```python
from build123d import *

# Parameters (mm, degrees)
F0_R     = 12.5
F1_DEPTH = 5
F2_R     = 6.5
F3_DEPTH = 2.54
F4_DEPTH = 3
F5_R     = 6.5
F6_DEPTH = 3


with BuildPart() as f1:
    # F0 (on Top) → F1 (new body)
    with BuildSketch(Plane.XY):
        Circle(F0_R)
    extrude(amount=F1_DEPTH)

    # F2 (on Top) → F3 (join)
    with BuildSketch(Plane.XY):
        Circle(F2_R)
    extrude(amount=F3_DEPTH)

    # F2 (on Top) → F4 (join)
    with BuildSketch(Plane.XY):
        Circle(F2_R)
    extrude(amount=F4_DEPTH)

    # F5 (on Top) → F6 (cut)
    with BuildSketch(Plane.XY):
        Circle(F5_R)
    extrude(amount=F6_DEPTH, mode=Mode.SUBTRACT)


solid = f1.part
```
The model under review builds one solid part; all positions refer to its coordinate system, in mm. A direction names the side the tool comes from. Round coordinates to 2 decimals unless told otherwise and drop trailing zeros. Write each loop counter-clockwise with the first axis right and the second up, starting at its lowest first coordinate (ties: lowest second). Pieces come first, ordered by that corner, then holes.
(1) Machinability: for faces 4 (the flat face through (0, 0, 5)), 5 (the cylindrical face through (-5.158, -3.955, 1.479)), which of the approach directions +Z, -Z, +X, -X, +Y, -Y give a long, thin tool a straight path to every point of the face, cutting with its end or side? Answer none if there is none.
(2) We need section D-D on z = 3.35. Give the boundary of the cut face in (x, y), and give its area (3 significant figures).
(3) Wall thickness on L1, parallel to Y at x = 0, z = 1.3; L2, parallel to Z at x = 5.25, y = -2; L3, parallel to X at y = 5.75, z = 2.5: over which ranges is each line inside the solid? List them lowest first.
(4) Mouldability with a two-part tool opening along X and no side actions: class faces 1 (the cylindrical face through (11.923, 3.755, 2.465)), 2 (the flat face through (0, 0, 3)), 3 (the flat face through (5, -5, 0)) as +X half, -X half, draft (parallel to the pull), parting line (faces both ways), or undercut.
(5) We need section C-C on z = 0.4. Give the boundary of the cut face in (x, y).
(6) Insertion check: pin 1 (3 mm diameter, centred on y = -6.5, z = 3.5, fed in from -X); pin 2 (3 mm diameter, centred on y = -3.5, z = 2.5, fed in from +X); pin 3 (4 mm diameter, centred on x = 0, y = 2.5, fed in from -Z). Each pin has a flat end and moves straight along its axis. Give the tip position at first contact, or say it passes through.
(7) We need section A-A on x = 0. Give the boundary of the cut face in (y, z), and give its area (3 significant figures).
Findings below:
1. face 4: +Z, +X, -X, +Y, -Y
1. face 5: -Z
2. outline: circle Ø25 at (0, 0)
2. area: 491 mm2
3. L1: y = -12.5 to -6.5, 6.5 to 12.5
3. L2: z = 3 to 5
3. L3: x = -11.1 to -3.03, 3.03 to 11.1
4. face 1: parting line
4. face 2: undercut
4. face 3: draft
5. outline: circle Ø25 at (0, 0); hole circle Ø13 at (0, 0)
6. pin 1: stops at x = -11.46
6. pin 2: stops at x = 12.34
6. pin 3: stops at z = 3
7. outline: (-12.5, 0) - (-6.5, 0) - (-6.5, 3) - (6.5, 3) - (6.5, 0) - (12.5, 0) - (12.5, 5) - (-12.5, 5) - close
7. area: 86.0 mm2
